```python
from build123d import *

# Parameters (mm, degrees)
SKETCH1_W               = 609.6
SKETCH1_H               = 609.6
BOSS_EXTRUDE1_DEPTH     = 304.8
CUT_EXTRUDE2_DEPTH      = 747.6044736
CUT_EXTRUDE2_DEPTH_BACK = 609.6
SHELL11_T               = -12.7
CUT_EXTRUDE5_REACH      = 645.809
SKETCH12_W              = 62.23
SKETCH12_H              = 75.184
CUT_EXTRUDE6_REACH      = 529.929
SKETCH13_W              = 152.4
SKETCH13_H              = 127
BOSS_EXTRUDE2_DEPTH     = 158.496
SHELL13_START           = -292.1
SHELL13_DEPTH           = 145.796
BOSS_EXTRUDE4_REACH     = 738.271
SKETCH16_W              = 123.026433271
SKETCH16_H              = 113.837135886
CUT_EXTRUDE7_DEPTH      = 158.496


# Read off the part's stored shape, not the designer's step: Shell13
with BuildPart() as part:
    # Sketch1 → Boss-Extrude1 (new body)
    with BuildSketch(Plane(origin=(0, 0, 0), x_dir=(1, 0, 0), z_dir=(0, 1, 0))):
        Rectangle(SKETCH1_W, SKETCH1_H)
    extrude(amount=BOSS_EXTRUDE1_DEPTH)

    # Sketch11 → Cut-Extrude2 (cut, two sides: drawn at the far end of the back side and taken through both)
    with BuildSketch(Plane(origin=(304.8, 0, 0), x_dir=(0, 0, -1), z_dir=(1, 0, 0)).offset(-CUT_EXTRUDE2_DEPTH_BACK)):
        Polygon((-1382.429640083, -515.219760055), (-304.8, 203.2), (-152.4, 304.8), (925.229640083, 1023.219760055), (-511.609880028, 3178.47904022), (-2819.269160193, 1640.03952011), align=None)
    extrude(amount=CUT_EXTRUDE2_DEPTH + CUT_EXTRUDE2_DEPTH_BACK, mode=Mode.SUBTRACT)

    # Shell11
    shell11_openings = [part.faces().sort_by_distance(p)[0] for p in [
        (0, 152.4, -304.8),
    ]]
    offset(amount=SHELL11_T, openings=shell11_openings, kind=Kind.INTERSECTION)

    # Sketch12 → Cut-Extrude5 (cut, up to next)
    with BuildSketch(Plane(origin=(0, 281.353846154, 187.569230769), x_dir=(1, 0, 0), z_dir=(0, 0.8320502943378435, 0.5547001962252293)), mode=Mode.PRIVATE) as cut_extrude5_sk1:
        with Locations((135.847083822, -49.312847444)):
            Rectangle(SKETCH12_W, SKETCH12_H)
    cut_extrude5_tool1 = extrude(cut_extrude5_sk1.sketch, amount=-CUT_EXTRUDE5_REACH, mode=Mode.PRIVATE) & part.part
    add(cut_extrude5_tool1.solids().sort_by_distance((135.847084, 254, 228.6))[0], mode=Mode.SUBTRACT)

    # Sketch13 → Cut-Extrude6 (cut, up to next)
    with BuildSketch(Plane(origin=(0, 304.8, 0), x_dir=(1, 0, 0), z_dir=(0, 1, 0)), mode=Mode.PRIVATE) as cut_extrude6_sk1:
        with Locations((-215.9, -76.2)):
            Rectangle(SKETCH13_W, SKETCH13_H)
    cut_extrude6_tool1 = extrude(cut_extrude6_sk1.sketch, amount=-CUT_EXTRUDE6_REACH, mode=Mode.PRIVATE) & part.part
    add(cut_extrude6_tool1.solids().sort_by_distance((-215.9, 304.8, 76.2))[0], mode=Mode.SUBTRACT)

    # Sketch14 → Boss-Extrude2 (add)
    with BuildSketch(Plane(origin=(-292.1, 0, 0), x_dir=(0, 0, -1), z_dir=(1, 0, 0))):
        Polygon((-292.1, 12.7), (-8.096776742, 12.7), (-8.096776742, 292.1), (-148.554749401, 292.1), (-292.1, 196.403166267), align=None)
    extrude(amount=BOSS_EXTRUDE2_DEPTH)

    # Shell13 outline → Shell13 (cut)
    with BuildSketch(Plane.YZ.offset(SHELL13_START)):
        Polygon((196.403166267, 292.1), (12.7, 292.1), (12.7, 20.796776742), (292.1, 20.796776742), (292.1, 148.554749401), align=None)
    extrude(amount=SHELL13_DEPTH, mode=Mode.SUBTRACT)

    # Sketch15 → Boss-Extrude4 (add, up to next)
    with BuildSketch(Plane(origin=(-292.1, 0, 0), x_dir=(0, 0, -1), z_dir=(1, 0, 0)), mode=Mode.PRIVATE) as boss_extrude4_sk1:
        Polygon((-292.1, 59.544316955), (-20.796776742, 166.882273248), (-20.796776742, 158.761495931), (-292.1, 51.423539637), align=None)
    boss_extrude4_tool1 = extrude(boss_extrude4_sk1.sketch, amount=BOSS_EXTRUDE4_REACH, mode=Mode.PRIVATE) - part.part
    add(boss_extrude4_tool1.solids().sort_by_distance((-292.1, 109.152906, 156.448388))[0])

    # Sketch16 → Cut-Extrude7 (cut)
    with BuildSketch(Plane(origin=(0, 0, 292.1), x_dir=(-1, 0, 0), z_dir=(0, 0, -1))):
        with Locations((217.055324109, 116.462884898)):
            Rectangle(SKETCH16_W, SKETCH16_H)
    extrude(amount=-CUT_EXTRUDE7_DEPTH, mode=Mode.SUBTRACT)


solid = part.part
```
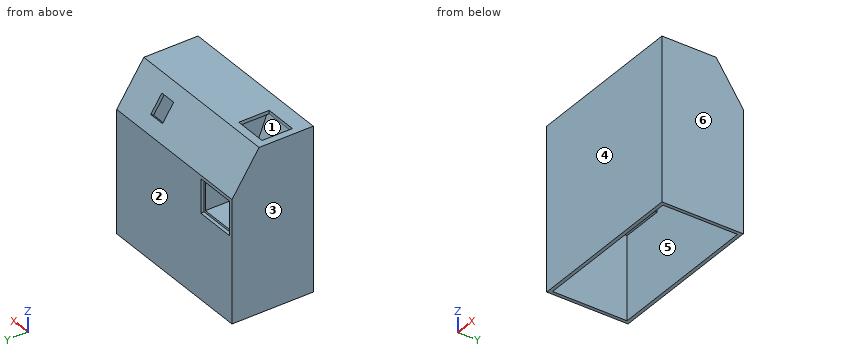
Can you work these out from the model? Positions are in its coordinate system, mm. Face numbers are marked on the shaded views. A direction names the side the tool comes from. Coordinates: 2 decimals unless noted, no trailing zeros. Loops run counter-clockwise (first coordinate to the right, second up) from the corner with the lowest first, then second, coordinate; pieces in that order, holes last. Notation, with made-up numbers: M 38,82 L 89,82 A13 ccw 89,92 Z; hole C 47.5,57.25 d11. An arc over 180 degrees is marked long. Put each result on its own line as item: value. Start each with the question number.
(1) Which directions (+Z, -Z, +X, -X, +Y, -Y) give clear straight access to the entire face, cutting with the end or side of a thin tool? Please do the marked faces 5 and 6.
(2) Will these pins go through, and if not, where does the flat tip stop? pin 1 Ø10 at (x, y) = (-233.5, 300) entering from +Z; pin 2 Ø10 at (x, z) = (-202, 298) entering from +Y; pin 3 Ø1.5 at (x, y) = (65.5, 112) entering from -Z.
(3) Imagine slicing it at C-C on x = 113. List the corners of the cut face in (y, z) for me.
(4) Imagine slicing it at A-A on x = -225.5. List the corners of the cut face in (y, z) for me, and give its area (3 significant figures).
(5) Imagine slicing it at D-D on y = 37. List the corners of the cut face in (x, z) for me.
(6) I need wall thicknesses on probe 1 along X at (y, z) = (188.5, 75.5); probe 2 along Y at (x, z) = (-132, -11); probe 3 along X at (y, z) = (88.5, -119). Which ranges of each line are inside material? Lowest first, please.
(7) Imagine slicing it at B-B on z = -47. List the corners of the cut face in (x, y) for me.
(8) We'd pull the mould along Y, two halves only. Please class the marked faces 1, 2, 3 and 4: +Y half, -Y half, draft (parallel to the pull), parting line (faces both ways), or undercut.
Worked answers:
1. face 5: -Z
1. face 6: +Z, -Z, +X, +Y, -Y
2. pin 1: stops at z = 167.1
2. pin 2: stops at y = 211.07
2. pin 3: stops at z = 292.1
3. outline: M 0,-304.8 L 12.7,-304.8 L 12.7,292.1 L 196.4,292.1 L 222.58,252.83 L 233.15,259.88 L 203.2,304.8 L 0,304.8 Z; M 264.29,190.28 L 292.1,148.55 L 292.1,-304.8 L 304.8,-304.8 L 304.8,152.4 L 274.85,197.32 Z
4. outline: M 0,-304.8 L 12.7,-304.8 L 12.7,8.1 L 292.1,8.1 L 292.1,-304.8 L 304.8,-304.8 L 304.8,12.7 L 292.1,12.7 L 292.1,20.8 L 166.88,20.8 L 59.54,292.1 L 59.54,304.8 L 0,304.8 Z; M 173.38,292.1 L 196.4,292.1 L 292.1,148.55 L 292.1,139.7 L 304.8,139.7 L 304.8,152.4 L 203.2,304.8 L 173.38,304.8 Z; hole M 12.7,20.8 L 158.76,20.8 L 51.42,292.1 L 12.7,292.1 Z
4. area: 20,900 mm2
5. outline: M -304.8,-304.8 L -292.1,-304.8 L -292.1,8.1 L -133.6,8.1 L -133.6,292.1 L 292.1,292.1 L 292.1,-304.8 L 304.8,-304.8 L 304.8,304.8 L -304.8,304.8 Z; hole M -292.1,20.8 L -146.3,20.8 L -146.3,292.1 L -292.1,292.1 Z
6. probe 1: x = -304.8 to -292.1, -146.3 to -133.6, 292.1 to 304.8
6. probe 2: y = 0 to 12.7, 292.1 to 304.8
6. probe 3: x = -304.8 to -292.1, 292.1 to 304.8
7. outline: M -304.8,0 L 304.8,0 L 304.8,304.8 L -304.8,304.8 Z; hole M -292.1,12.7 L 292.1,12.7 L 292.1,292.1 L -292.1,292.1 Z
8. face 1: undercut
8. face 2: +Y half
8. face 3: draft
8. face 4: -Y half
